Design review of the part built by this model. Coordinates are the model's own, in mm. A direction names the side the tool comes from. Give positions to 0.01 mm unless a question says otherwise; leave off trailing zeros. Loops run counter-clockwise (first coordinate to the right, second up) from the corner with the lowest first, then second, coordinate; pieces in that order, holes last. Notation, with made-up numbers: M 86.5,36.25 L 111.5,36.25 A24 ccw 111.5,74.25 Z; hole C -18,60 d3. An arc over 180 degrees is marked long. Use CSV: the item, a comma, the result in double quotes.
from build123d import *

# Parameters (mm, degrees)
SKETCH1_W             = 45
SKETCH1_H             = 40
PCB_DEPTH             = 1.6
SKETCH2_W             = 10.5
SKETCH2_H             = 30
MOTOR_TERMINALS_DEPTH = 10.4
SKETCH3_W             = 10.5
SKETCH3_H             = 16
POWER_TERMINAL_DEPTH  = 10.4


with BuildPart() as part:
    # Sketch1 → PCB (new body)
    with BuildSketch(Plane.XY):
        Rectangle(SKETCH1_W, SKETCH1_H)
    extrude(amount=PCB_DEPTH)

    # Sketch2 → Motor_terminals (add)
    with BuildSketch(Plane.XY.offset(1.6)):
        with Locations((-17.25, 0)):
            Rectangle(SKETCH2_W, SKETCH2_H)
    extrude(amount=MOTOR_TERMINALS_DEPTH)

    # Sketch3 → Power_terminal (add)
    with BuildSketch(Plane.XY.offset(1.6)):
        with Locations((17.25, 0)):
            Rectangle(SKETCH3_W, SKETCH3_H)
    extrude(amount=POWER_TERMINAL_DEPTH)


solid = part.part
(1) We need section C-C on x = 17. State the section outline as (y, z) points, then the cut area to 3 significant figures.
A:
outline,"M -20,0 L 20,0 L 20,1.6 L 8,1.6 L 8,12 L -8,12 L -8,1.6 L -20,1.6 Z"
area,"230 mm²"
(2) The part is to be moulded in two halves that separate along X. For faces 1 (the flat face through (0, -20, 1)), 2 (the flat face through (12, 0, 7)), 3 (the flat face through (22.5, 0, 5)), say which applies: released by +X, released by -X, zero draft, split by the parting line, or undercut.
A:
face 1,"zero draft"
face 2,"undercut"
face 3,"released by +X"
(3) Clearance check with flat-ended pins moving along their axes: P1, Ø2, axis at x = 10, y = -6.5, coming from the +Z side; P2, Ø3, axis at x = -17.5, z = 9, coming from the +Y side; P3, Ø5, axis at x = 19, z = 5, coming from the -Y side. State where each tip first meets the part, or that it passes through.
A:
P1,"z = 1.6"
P2,"y = 15"
P3,"y = -8"
(4) Wall thickness on line 1 along X through (y, z) = (-4, 9.75); line 2 along X through (y, z) = (-12, 2.5); line 3 along Z through (x, y) = (11, -10): over which ranges is each line inside the solid? List them lowest first. Write a range as [from, to].
A:
line 1,"[-22.5, -12], [12, 22.5]"
line 2,"[-22.5, -12]"
line 3,"[0, 1.6]"
(5) We need section A-A on z = 2.25. State the section outline as (x, y) points, then the cut area to 3 significant figures.
A:
outline,"M -22.5,-15 L -12,-15 L -12,15 L -22.5,15 Z; M 12,-8 L 22.5,-8 L 22.5,8 L 12,8 Z"
area,"483 mm²"
(6) We need section D-D on y = 0. State the section outline as (x, z) points.
A:
outline,"M -22.5,0 L 22.5,0 L 22.5,12 L 12,12 L 12,1.6 L -12,1.6 L -12,12 L -22.5,12 Z"
(7) We need section B-B on y = -10. State the section outline as (x, z) points.
A:
outline,"M -22.5,0 L 22.5,0 L 22.5,1.6 L -12,1.6 L -12,12 L -22.5,12 Z"
(8) Machinability: for faces 4 (the flat face through (17, -8, 7)), 5 (the flat face through (-17, -15, 7)), 6 (the flat face through (-12, 0, 7)), 7 (the flat face through (-17, 15, 7)), 8 (the flat face through (17, 8, 7)), which of the approach directions +Z, -Z, +X, -X, +Y, -Y give a long, thin tool a straight path to every point of the face, cutting with its end or side? Answer none if there is none.
A:
face 4,"+Z, +X, -Y"
face 5,"+Z, +X, -X, -Y"
face 6,"+Z, +Y, -Y"
face 7,"+Z, +X, -X, +Y"
face 8,"+Z, +X, +Y"
